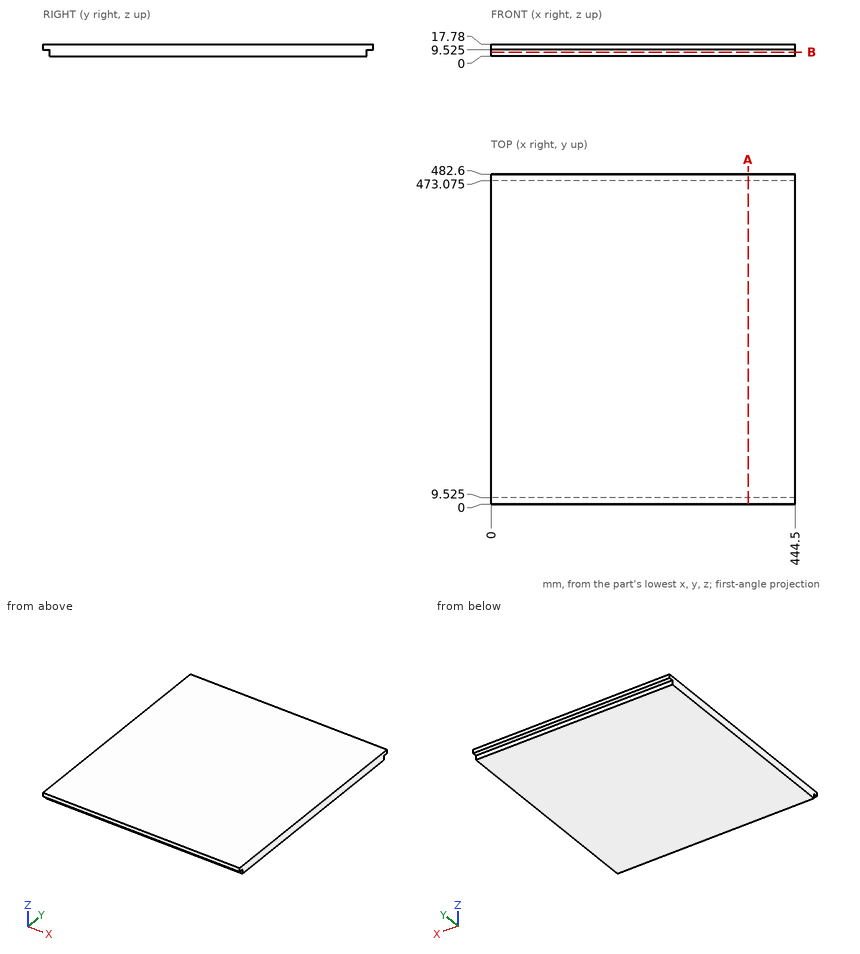
Could you check a few things on this drawing? It's one solid part, dimensions in mm from its lowest x, y, z. Coordinates: 2 decimals unless noted, no trailing zeros. Order: outer loops, then holes, each group sorted by start corner. A loop starts at its lowest first (then second) coordinate and runs counter-clockwise, first axis right, second up. Notation, with made-up numbers: M 58.25,-25 L 71.25,-25 A27 cw 71.25,-5 Z; hole C 47.5,37.25 d8. An arc over 180 degrees is marked long. Answer as a JSON object with one key per item and string values. Group by question number.
(1) Suppose I cut it at A-A, the plane x = 376. Please give me the cut outline in (y, z) (3 decimals), then the cut area to 3 significant figures.
(2) Suppose I cut it at B-B, the plane z = 6. Please give me the cut outline in (x, y) (3 decimals), then the cut area to 3 significant figures.
(3) I need wall thicknesses on probe 1 along Y at (x, z) = (418, 7.5) (3 decimals). Which ranges of the line are inside material? Lowest first, please.
(4) For pin 1 (3 mm diameter, centred on x = 289, y = 477.5, fed in from -Z) (3 decimals); pin 2 (7.5 mm diameter, centred on x = 171.5, z = 5, fed in from +Y) (3 decimals), each with a flat end and sliding along its axis, tell me the tip position at first contact or that it passes through.
Values found:
{
 "1": {"outline": "M 0,9.525 L 9.525,9.525 L 9.525,0 L 473.075,0 L 473.075,9.525 L 482.6,9.525 L 482.6,17.78 L 0,17.78 Z", "area": "8,400 mm^2"},
 "2": {"outline": "M 0,9.525 L 444.5,9.525 L 444.5,473.075 L 0,473.075 Z", "area": "206,000 mm^2"},
 "3": {"probe 1": "y = 9.525 to 473.075"},
 "4": {"pin 1": "stops at z = 9.525", "pin 2": "stops at y = 473.075"}
}
